Design review of the part built by this model. Coordinates are the model's own, in mm. A direction names the side the tool comes from. Coordinates: 2 decimals unless noted, no trailing zeros. Order: outer loops, then holes, each group sorted by start corner. A loop starts at its lowest first (then second) coordinate and runs counter-clockwise, first axis right, second up. Notation, with made-up numbers: (-13, 57) -> (5, 57) arc R15 cw to (5, 86) -> close; hole circle Ø4 at (53.25, -10). An arc over 180 degrees is marked (long way). Use a Markdown table: item, result. Add a question column.
Q1. Machinability: for faces 1 (the face through (6.6, 0.8, 94.4)), 2 (the face through (6, 1.5, 56)), 3 (the face through (6, 0, 56)), which of the approach directions +Z, -Z, +X, -X, +Y, -Y give a long, thin tool a straight path to every point of the face, cutting with its end or side? Answer none if there is none.
Q2. Add section B-B (z = 24.4). State the section outline as (x, y) points, then the cut area to 3 significant figures.
Q3. Add section D-D (y = 47.1). State the section outline as (x, z) points, then the cut area to 3 significant figures.
Q4. Add section A-A (y = 26.7). State the section outline as (x, z) points, then the cut area to 3 significant figures.
Q5. Insertion check: pin 1 (3 mm diameter, centred on y = 26.7, z = 98.8, fed in from -X); pin 2 (1.2 mm diameter, centred on y = 1, z = 26.5, fed in from -X); pin 3 (5.5 mm diameter, centred on y = 41.7, z = 32.2, fed in from +X); pin 4 (1.2 mm diameter, centred on y = 0.5, z = 87.5, fed in from -X). Each pin has a flat end and moves straight along its axis. Give the tip position at first contact, or say it passes through.
Q6. Add section C-C (z = 80). State the section outline as (x, y) points, then the cut area to 3 significant figures.
Q7. Wall thickness on probe 1 along Y at (x, z) = (0.7, 98.8); probe 2 along Y at (x, z) = (0.8, 32.2); probe 3 along Z at (x, y) = (1.2, 68.5): over which ranges is each line inside the solid? List them lowest first.
Q8. The part is to be moulded in two halves that separate along X. For faces 4 (the face through (0.64, 0.67, 55.82)), 5 (the face through (0.74, 42.226, 18.269)), 6 (the face through (6.6, 0.8, 35.2)), say which applies: pulls with the +X half, pulls with the -X half, needs draft (parallel to the pull), parting line crosses it, or undercut.
from build123d import *

# Parameters (mm, degrees)
SKETCH_1_W                       = 1.5
SKETCH_1_H                       = 90
SM_BASE_FLANGE_1_DEPTH           = 110.1
SKETCH_6_R                       = 7
SKETCH_6_R_2                     = 1.75
CUT_EXTRUDE_1_DEPTH              = 10
SM_EDGE_FLANGE_1_STRIP_W         = 7.4732
SM_EDGE_FLANGE_1_STRIP_H         = 1.5
SM_EDGE_FLANGE_1_STRIP_CUT_DEPTH = 110.1
SM_EDGE_FLANGE_1_DEPTH           = 110.1
CUT_EXTRUDE_2_DEPTH              = 10


# Sheet-metal steps are written as plain solids
with BuildPart() as part:
    # Sketch 1 → 基体-法兰1 (new body)
    with BuildSketch(Plane.XY):
        with Locations((0.75, 45)):
            Rectangle(SKETCH_1_W, SKETCH_1_H)
    extrude(amount=SM_BASE_FLANGE_1_DEPTH)

    # 草图6 → 切除-拉伸1 (cut)
    with BuildSketch(Plane.ZY):
        with Locations((24.4, 62.1)):
            Circle(SKETCH_6_R)
        with Locations((91, 47.1)):
            Circle(SKETCH_6_R)
        with Locations((16.6, 68.5)):
            Circle(SKETCH_6_R_2)
        with Locations((16.6, 41.7)):
            Circle(SKETCH_6_R_2)
        with Locations((32.2, 41.7)):
            Circle(SKETCH_6_R_2)
        with Locations((32.2, 68.5)):
            Circle(SKETCH_6_R_2)
        with Locations((83.2, 53.5)):
            Circle(SKETCH_6_R_2)
        with Locations((83.2, 26.7)):
            Circle(SKETCH_6_R_2)
        with Locations((98.8, 26.7)):
            Circle(SKETCH_6_R_2)
        with Locations((98.8, 53.5)):
            Circle(SKETCH_6_R_2)
    extrude(amount=-CUT_EXTRUDE_1_DEPTH, mode=Mode.SUBTRACT)

    # 边线-法兰1 strip (across the edge) → 边线-法兰1 strip cut (cut)
    with BuildSketch(Plane(origin=(1.5, 0, 110.1), x_dir=(0, 1, 0), z_dir=(0, 0, -1))):
        with Locations((-1.5, -0.75)):
            Rectangle(SM_EDGE_FLANGE_1_STRIP_W, SM_EDGE_FLANGE_1_STRIP_H)
    extrude(amount=SM_EDGE_FLANGE_1_STRIP_CUT_DEPTH, mode=Mode.SUBTRACT)

    # 边线-法兰1 section (across the edge) → 边线-法兰1 (add)
    with BuildSketch(Plane(origin=(1.5, 0, 110.1), x_dir=(0, 1, 0), z_dir=(0, 0, -1))):
        with BuildLine():
            Line((0, 0.7366), (0, 8.5))
            Line((0, 8.5), (1.5, 8.5))
            Line((1.5, 8.5), (1.5, 0.7366))
            ThreePointArc((1.5, 0.7366), (1.715745145, 0.215745145), (2.2366, 0))
            Line((2.2366, 0), (2.2366, -1.5))
            ThreePointArc((2.2366, -1.5), (0.655084973, -0.844915027), (0, 0.7366))
        make_face()
    extrude(amount=SM_EDGE_FLANGE_1_DEPTH)

    # 草图10 → 切除-拉伸2 (cut)
    with BuildSketch(Plane(origin=(0, 1.5, 0), x_dir=(1, 0, 0), z_dir=(0, 1, 0))):
        with BuildLine():
            Line((8.85, -17.95), (8.85, -32.95))
            ThreePointArc((8.85, -32.95), (6.6, -35.2), (4.35, -32.95))
            Line((4.35, -32.95), (4.35, -17.95))
            ThreePointArc((4.35, -17.95), (6.6, -15.700000154), (8.85, -17.95))
        make_face()
        with BuildLine():
            Line((4.35, -92.15), (4.35, -77.15))
            ThreePointArc((4.35, -77.15), (6.6, -74.899999913), (8.85, -77.15))
            Line((8.85, -77.15), (8.85, -92.15))
            ThreePointArc((8.85, -92.15), (6.6, -94.4), (4.35, -92.15))
        make_face()
    extrude(amount=-CUT_EXTRUDE_2_DEPTH, mode=Mode.SUBTRACT)


solid = part.part
Established:
| question | item | result |
|---|---|---|
| 1 | face 1 | +Y, -Y |
| 1 | face 2 | +Z, -Z, +X, +Y |
| 1 | face 3 | +Z, -Z, +X, -X, -Y |
| 2 | outline | (0, 2.24) arc R2.24 ccw to (2.24, 0) -> (4.35, 0) -> (4.35, 1.5) -> (2.24, 1.5) arc R0.74 cw to (1.5, 2.24) -> (1.5, 55.1) -> (0, 55.1) -> close; (0, 69.1) -> (1.5, 69.1) -> (1.5, 90) -> (0, 90) -> close; (8.85, 0) -> (10, 0) -> (10, 1.5) -> (8.85, 1.5) -> close |
| 2 | area | 119 mm^2 |
| 3 | outline | (0, 0) -> (1.5, 0) -> (1.5, 84) -> (0, 84) -> close; (0, 98) -> (1.5, 98) -> (1.5, 110.1) -> (0, 110.1) -> close |
| 3 | area | 144 mm^2 |
| 4 | outline | (0, 0) -> (1.5, 0) -> (1.5, 81.45) -> (0, 81.45) -> close; (0, 84.95) -> (1.5, 84.95) -> (1.5, 97.05) -> (0, 97.05) -> close; (0, 100.55) -> (1.5, 100.55) -> (1.5, 110.1) -> (0, 110.1) -> close |
| 4 | area | 155 mm^2 |
| 5 | pin 1 | through |
| 5 | pin 2 | x = 0.09 |
| 5 | pin 3 | x = 1.5 |
| 5 | pin 4 | x = 0.31 |
| 6 | outline | (0, 2.24) arc R2.24 ccw to (2.24, 0) -> (4.35, 0) -> (4.35, 1.5) -> (2.24, 1.5) arc R0.74 cw to (1.5, 2.24) -> (1.5, 90) -> (0, 90) -> close; (8.85, 0) -> (10, 0) -> (10, 1.5) -> (8.85, 1.5) -> close |
| 6 | area | 140 mm^2 |
| 7 | probe 1 | 0.61 to 24.95, 28.45 to 51.75, 55.25 to 90 |
| 7 | probe 2 | 0.52 to 39.95, 43.45 to 66.75, 70.25 to 90 |
| 7 | probe 3 | 0 to 14.85, 18.35 to 21.56, 27.24 to 30.45, 33.95 to 110.1 |
| 8 | face 4 | pulls with the -X half |
| 8 | face 5 | needs draft |
| 8 | face 6 | undercut |
